Can you work these out from the model? Positions are in its coordinate system, mm. Face numbers are marked on the shaded views. Round coordinates to 2 decimals unless told otherwise and drop trailing zeros. Order: outer loops, then holes, each group sorted by start corner. A loop starts at its lowest first (then second) coordinate and runs counter-clockwise, first axis right, second up. Notation, with made-up numbers: (82, -24) -> (100, -24) arc R15 ccw to (100, -13) -> close; hole circle Ø2 at (55, 41.25). An arc over 180 degrees is marked (long way). Use a Markdown table: item, result. Add a question column.
Q1. If we section it at B-B on y = 1.45: List the corners of the cut face in (x, z) for me, plus the area to 3 significant figures.
Q2. We'd pull the mould along Z, two halves only. Please class the marked faces 1 and 2: +Z half, -Z half, draft (parallel to the pull), parting line (faces both ways), or undercut.
Q3. I need wall thicknesses on line 1 along X through (y, z) = (2.5, 6); line 2 along X through (y, z) = (2.45, 4); line 3 along Z through (x, y) = (-0.5, 0.4). Which ranges of each line are inside material? Lowest first, please. Write a range as [from, to].
Q4. I'm going to push flat-ended pins straight in: pin 1 Ø3 at (x, z) = (0.5, 0) entering from -Y; pin 2 Ø1 at (y, z) = (0.5, 4) entering from -X; pin 3 Ø0.7 at (y, z) = (2.5, -3.5) entering from +X; pin 4 Ø0.7 at (x, y) = (2, 2) entering from -Z. Where does each tip first touch, or does it pass through?
Q5. If we section it at C-C on x = 7: List the corners of the cut face in (y, z) for me (3 decimals), plus the area to 3 significant figures.
Q6. If we section it at A-A on z = 1.5: List the corners of the cut face in (x, y) for me.
Q7. If we section it at D-D on x = 1: List the corners of the cut face in (y, z) for me, plus the area to 3 significant figures.
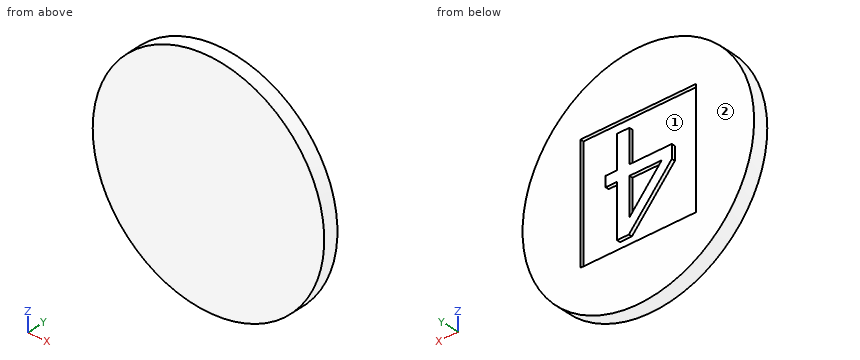
Autodesk Inventor part; units mm, degrees
ref_plane "YZ Plane" through (0, 0, 0) normal (1, 0, 0) x (0, 1, 0)
ref_plane "XZ Plane" through (0, 0, 0) normal (0, 1, 0) x (-1, 0, 0)
ref_plane "XY Plane" through (0, 0, 0) normal (0, 0, 1) x (1, 0, 0)
sketch "Sketch1" plane through (0, 0, 0) normal (0, 1, 0) x (-1, 0, 0)
  circle A0 centre (0, 0) radius 20
  dimension "d0" = 40
extrude "Extrusion1" add sketch "Sketch1" along normal blind 2.6
sketch "Sketch2" plane through (0, 2.6, 0) normal (0, 1, 0) x (1, 0, 0)
  line L0 (-10, -10) -> (-10, 10)
  line L1 (-10, 10) -> (10, 10)
  line L2 (10, 10) -> (10, -10)
  line L3 (10, -10) -> (-10, -10)
  line L4 (-10, -10) -> (10, 10) construction
  line L5 (-10, 10) -> (10, -10) construction
  point P0 (0, 0)
  dimension "d3" = 20
  dimension "d4" = 20
extrude "Extrusion2" cut sketch "Sketch2" against normal blind 0.6
sketch "Sketch3" plane through (0, 2, 0) normal (0, 1, 0) x (1, 0, 0)
  line L0 (-6.2284, 8.4382) -> (6.2284, 8.4382) construction
  line L1 (6.2284, 8.4382) -> (6.2284, -8.1618) construction
  line L2 (6.2284, -8.1618) -> (-6.2284, -8.1618) construction
  line L3 (-6.2284, -8.1618) -> (-6.2284, 8.4382) construction
  line L4 (5.6634, -2.4581) -> (3.6859, -2.4581)
  line L5 (3.6859, -2.4581) -> (3.6859, -8.1618)
  line L6 (3.6859, -8.1618) -> (1.547, -8.1618)
  line L7 (1.547, -8.1618) -> (1.547, -2.4581)
  line L8 (1.547, -2.4581) -> (-5.7844, -2.4581)
  line L9 (-5.7844, -2.4581) -> (-5.7844, -0.1174)
  line L10 (-5.7844, -0.1174) -> (1.6412, 8.4382)
  line L11 (1.6412, 8.4382) -> (3.6859, 8.4382)
  line L12 (3.6859, 8.4382) -> (3.6859, -0.6689)
  line L13 (3.6859, -0.6689) -> (5.6634, -0.6689)
  line L14 (5.6634, -0.6689) -> (5.6634, -2.4581)
  line L15 (1.547, -0.6689) -> (1.547, 5.815)
  line L16 (1.547, 5.815) -> (-4.0357, -0.6689)
  line L17 (-4.0357, -0.6689) -> (1.547, -0.6689)
  point P0 (0, 0)
extrude "Extrusion3" add sketch "Sketch3" along normal blind 0.6
properties part number "TopMarker4"
Answer below:
| question | item | result |
|---|---|---|
| 1 | outline | circle Ø40 at (0, 0) |
| 1 | area | 1,260 mm² |
| 2 | face 1 | undercut |
| 2 | face 2 | draft |
| 3 | line 1 | [-19.08, -10], [1.55, 3.69], [10, 19.08] |
| 3 | line 2 | [-19.6, -10], [1.55, 3.69], [10, 19.6] |
| 3 | line 3 | [-19.99, 19.99] |
| 4 | pin 1 | y = 0 |
| 4 | pin 2 | x = -19.69 |
| 4 | pin 3 | x = 19.75 |
| 4 | pin 4 | z = -19.93 |
| 5 | outline | (0, -18.735) -> (2.6, -18.735) -> (2.6, -10) -> (2, -10) -> (2, 10) -> (2.6, 10) -> (2.6, 18.735) -> (0, 18.735) -> close |
| 5 | area | 85.4 mm² |
| 6 | outline | (-19.94, 0) -> (19.94, 0) -> (19.94, 2.6) -> (10, 2.6) -> (10, 2) -> (5.66, 2) -> (5.66, 2.6) -> (-5.78, 2.6) -> (-5.78, 2) -> (-10, 2) -> (-10, 2.6) -> (-19.94, 2.6) -> close |
| 7 | outline | (0, -19.97) -> (2.6, -19.97) -> (2.6, -10) -> (2, -10) -> (2, -7.7) -> (2.6, -7.7) -> (2.6, -5.18) -> (2, -5.18) -> (2, 0.67) -> (2.6, 0.67) -> (2.6, 2.46) -> (2, 2.46) -> (2, 10) -> (2.6, 10) -> (2.6, 19.97) -> (0, 19.97) -> close |
| 7 | area | 94.5 mm² |
